from build123d import *

# Parameters (mm, degrees)
F1_DEPTH  = 76.2
F5_DEPTH  = 25.4
F8_DEPTH  = 25.4
F10_W     = 457.2
F10_H     = 431.8
F10_W_2   = 419.1
F10_H_2   = 187.325
F11_DEPTH = 431.8
F12_W     = 76.2
F12_H     = 25.4
F13_DEPTH = 508


with BuildPart() as f1:
    # F0 (on Top) → F1 (new body)
    with BuildSketch(Plane.XY):
        Polygon((228.6, -228.6), (254, -228.6), (254, 228.6), (-254, 228.6), (-254, -228.6), (-228.6, -228.6), (-228.6, 203.2), (229.069446, 203.2), align=None)
    extrude(amount=F1_DEPTH)

    # F4 (on offset) → F5 (join)
    with BuildSketch(Plane.YZ.offset(254)):
        Polygon((123.634481, 76.2), (228.6, 76.2), (-152.4, 478.366667), (-152.4, 1244.6), (-228.6, 1244.6), (-228.6, 448.003064), align=None)
    extrude(amount=-F5_DEPTH)

    # F7 (on offset) → F8 (join)
    with BuildSketch(Plane.YZ.offset(-254)):
        Polygon((123.634481, 76.2), (228.6, 76.2), (-152.4, 478.366667), (-152.4, 1244.6), (-228.6, 1244.6), (-228.6, 448.003064), align=None)
    extrude(amount=F8_DEPTH)

    # F10 (on offset) → F11 (join)
    with BuildSketch(Plane.XZ.offset(228.6)):
        with Locations((0, 1054.1)):
            Rectangle(F10_W, F10_H)
        with Locations((0, 950.9125)):
            Rectangle(F10_W_2, F10_H_2, mode=Mode.SUBTRACT)
        with Locations((0, 1157.2875)):
            Rectangle(F10_W_2, F10_H_2, mode=Mode.SUBTRACT)
    extrude(amount=-F11_DEPTH)

    # F12 (on offset) → F13 (join)
    with BuildSketch(Plane.YZ.offset(254)):
        with Locations((-190.5, 1257.3)):
            Rectangle(F12_W, F12_H)
    extrude(amount=-F13_DEPTH)


solid = f1.part
Can you work these out from the model? Positions are in its coordinate system, mm. A direction names the side the tool comes from. Coordinates: 2 decimals unless noted, no trailing zeros. Loops run counter-clockwise (first coordinate to the right, second up) from the corner with the lowest first, then second, coordinate; pieces in that order, holes last. Notation, with made-up numbers: (76, 50.25) - (135, 50.25) arc R26 cw to (135, 88.25) - close; hole circle Ø2 at (21.5, 65.5). An arc over 180 degrees is marked (long way). Put each result on its own line as item: value. Start each with the question number.
Item 1: Suppose I cut it at D-D (y = 52.5). Please give me the cut outline in (x, z) (3 decimals), and give its area (3 significant figures).
Item 2: Suppose I cut it at C-C (x = 3). Please give me the cut outline in (y, z) (3 decimals).
Item 3: Suppose I cut it at A-A (y = -101.5). Please give me the cut outline in (x, z) (3 decimals).
Item 4: For pin 1 (12.5 mm diameter, centred on x = -246, y = -82.5, fed in from +Z); pin 2 (23 mm diameter, centred on x = -65.5, y = -186, fed in from -Z); pin 3 (10 mm diameter, centred on x = 144.5, z = 1046, fed in from +Y), each with a flat end and sliding along its axis, tell me the tip position at first contact or that it passes through.
Item 5: If I drill on line 1 along Z through (x, y) = (169.5, 96) (3 decimals); line 2 along X through (y, z) = (170.5, 1030); line 3 along Z through (x, y) = (216, -157.5), over which ranges is the centre line in solid material (lowest first)?
Item 6: Which directions (+Z, -Z, +X, -X, +Y, -Y) give clear straight access to the entire face, cutting with the end or side of a thin tool? Please do faces 5 (the face through (-241, -152.4, 869)), 6 (the face through (-241.478, -54.948, 264.704)), 7 (the face through (4, 228.6, 38)), 8 (the face through (241, -152.4, 869)), 9 (the face through (209.55, -16, 950)).
Item 7: If we mould it in two halves opening along X, with no side actions, what happens to faces 1 (the face through (228.6, 23, 1051)), 2 (the face through (228.6, -120, 431)), 3 (the face through (-228.6, -69, 328)), 4 (the face through (-1, 203.2, 1055))? For each: +X half, -X half, draft (parallel to the pull), parting line (faces both ways), or undercut.
Item 8: Suppose I cut it at B-B (z = 788). Please give me the cut outline in (x, y).
Here are the results:
1. outline: (-254, 0) - (-228.6, 0) - (-228.6, 76.2) - (-254, 76.2) - close; (-254, 151.286) - (-228.6, 151.286) - (-228.6, 262.083) - (-254, 262.083) - close; (-228.6, 838.2) - (228.6, 838.2) - (228.6, 1270) - (-228.6, 1270) - close; (228.6, 151.286) - (254, 151.286) - (254, 262.083) - (228.6, 262.083) - close; (228.906, 0) - (254, 0) - (254, 76.2) - (228.906, 76.2) - close; hole (-209.55, 857.25) - (209.55, 857.25) - (209.55, 1044.575) - (-209.55, 1044.575) - close; hole (-209.55, 1063.625) - (209.55, 1063.625) - (209.55, 1250.95) - (-209.55, 1250.95) - close
1. area: 49,900 mm²
2. outline: (-228.6, 838.2) - (203.2, 838.2) - (203.2, 857.25) - (-228.6, 857.25) - close; (-228.6, 1044.575) - (203.2, 1044.575) - (203.2, 1063.625) - (-228.6, 1063.625) - close; (-228.6, 1244.6) - (-152.4, 1244.6) - (-152.4, 1250.95) - (203.2, 1250.95) - (203.2, 1270) - (-228.6, 1270) - close; (203.2, 0) - (228.6, 0) - (228.6, 76.2) - (203.2, 76.2) - close
3. outline: (-254, 0) - (-228.6, 0) - (-228.6, 76.2) - (-254, 76.2) - close; (-254, 313.842) - (-228.6, 313.842) - (-228.6, 424.639) - (-254, 424.639) - close; (-228.6, 838.2) - (228.6, 838.2) - (228.6, 1270) - (-228.6, 1270) - close; (228.6, 313.842) - (254, 313.842) - (254, 424.639) - (228.6, 424.639) - close; (228.738, 0) - (254, 0) - (254, 76.2) - (228.738, 76.2) - close; hole (-209.55, 857.25) - (209.55, 857.25) - (209.55, 1044.575) - (-209.55, 1044.575) - close; hole (-209.55, 1063.625) - (209.55, 1063.625) - (209.55, 1250.95) - (-209.55, 1250.95) - close
4. pin 1: z = 411.18
4. pin 2: z = 838.2
4. pin 3: y = 203.2
5. line 1: 838.2 to 857.25, 1044.575 to 1063.625, 1250.95 to 1270
5. line 2: -228.6 to -209.55, 209.55 to 228.6
5. line 3: 838.2 to 1270
6. face 5: +Z, -X, +Y
6. face 6: +X, -X, -Y
6. face 7: +Z, -Z, +X, -X, +Y
6. face 8: +Z, +X, +Y
6. face 9: +Y, -Y
7. face 1: +X half
7. face 2: undercut
7. face 3: undercut
7. face 4: draft
8. outline: (-254, -228.6) - (-228.6, -228.6) - (-228.6, -152.4) - (-254, -152.4) - close; (228.6, -228.6) - (254, -228.6) - (254, -152.4) - (228.6, -152.4) - close
